The listing builds one solid part. Answer for the finished solid, in the listing's coordinates (mm). A direction names the side the tool comes from. Coordinates: 2 decimals unless noted, no trailing zeros. Loops run counter-clockwise (first coordinate to the right, second up) from the corner with the lowest first, then second, coordinate; pieces in that order, holes last. Notation, with made-up numbers: (43, 38) - (89, 38) arc R12 ccw to (89, 49) - close; hole circle Ø7 at (-8, -31.75). An arc over 180 degrees is marked (long way). Put each result on its own line as item: value.
```python
from build123d import *

# Parameters (mm, degrees)
F0_R     = 40.64
F0_R_2   = 33.02
F1_DEPTH = 152.4
F2_R     = 76.2
F3_DEPTH = 25.4
F4_R     = 5.08
F5_R     = 5.08


with BuildPart() as f1:
    # F0 (on Front) → F1 (new body)
    with BuildSketch(Plane.XZ):
        Circle(F0_R)
        Circle(F0_R_2, mode=Mode.SUBTRACT)
    extrude(amount=F1_DEPTH)

    # F2 (on Front) → F3 (join)
    with BuildSketch(Plane.XZ):
        Circle(F2_R)
    extrude(amount=-F3_DEPTH)

    # F4
    f4_edges = [f1.edges().sort_by_distance(p)[0] for p in [
        (76.2, 12.7, 0),
        (-76.2, 0, 0),
        (-76.2, 25.4, 0),
    ]]
    fillet(f4_edges, radius=F4_R)

    # F5
    f5_edges = [f1.edges().sort_by_distance(p)[0] for p in [
        (-40.64, -152.4, 0),
    ]]
    fillet(f5_edges, radius=F5_R)


solid = f1.part
```
1) Straight lines are drawn through the part: L1, parallel to Z at x = 0, y = -114; L2, parallel to Y at x = -10, z = -23.5; L3, parallel to Z at x = -6.5, y = -91.5. For each, find the intervals that lie inside material, in ascending order. Write a range as [from, to].
Found:
L1: z = [-40.64, -33.02], [33.02, 40.64]
L2: y = [0, 25.4]
L3: z = [-40.12, -32.37], [32.37, 40.12]
2) The part is cut by section B-B (z = 0). Give the vertices of the cut face in (x, y).
Found:
outline: (-76.2, 5.08) arc R5.08 ccw to (-71.12, 0) - (-40.64, 0) - (-40.64, -147.32) arc R5.08 ccw to (-35.56, -152.4) - (-33.02, -152.4) - (-33.02, 0) - (33.02, 0) - (33.02, -152.4) - (35.56, -152.4) arc R5.08 ccw to (40.64, -147.32) - (40.64, 0) - (71.12, 0) arc R5.08 ccw to (76.2, 5.08) - (76.2, 20.32) arc R5.08 ccw to (71.12, 25.4) - (-71.12, 25.4) arc R5.08 ccw to (-76.2, 20.32) - close
3) The part is cut by section C-C (y = -55.5). Give the vertices of the cut face in (x, z).
Found:
outline: circle Ø81.28 at (0, 0); hole circle Ø66.04 at (0, 0)
4) For a pull along Z with two mould halves and no side action, classify faces 1 (the face through (-60.47, 12.593, -46.367)), 2 (the face through (31.5, -75.1, 9.9)), 3 (the face through (31, 0, -31)) as pulls with the +Z half, pulls with the -Z half, needs draft (parallel to the pull), parting line crosses it, or undercut.
Found:
face 1: parting line crosses it
face 2: undercut
face 3: needs draft
5) The part is cut by section D-D (y = 14). Give the vertices of the cut face in (x, z), and give its area (3 significant figures).
Found:
outline: circle Ø152.4 at (0, 0)
area: 18,200 mm^2
6) For faces 4 (the face through (-1, 25.4, 1)), 5 (the face through (0, 0, 0)), determine the directions among +Z, -Z, +X, -X, +Y, -Y from which every point of the face is accessible in a straight line to the end or side of a thin tool.
Found:
face 4: +Z, -Z, +X, -X, +Y
face 5: -Y
7) Each of these flat-tipped pins is pushed along its axis until it touches: pin 1 (3 mm diameter, centred on x = -21.5, y = -19, fed in from +Z); pin 2 (10 mm diameter, centred on x = -59.5, z = 36, fed in from -Y); pin 3 (8 mm diameter, centred on y = -94, z = -14.5, fed in from -X). Where does it stop, or does it pass through?
Found:
pin 1: stops at z = 35.38
pin 2: stops at y = 0
pin 3: stops at x = -39.26
8) The part is cut by section A-A (x = 0). Give the vertices of the cut face in (y, z), and give its area (3 significant figures).
Found:
outline: (-152.4, -35.56) arc R5.08 ccw to (-147.32, -40.64) - (0, -40.64) - (0, -71.12) arc R5.08 ccw to (5.08, -76.2) - (20.32, -76.2) arc R5.08 ccw to (25.4, -71.12) - (25.4, 71.12) arc R5.08 ccw to (20.32, 76.2) - (5.08, 76.2) arc R5.08 ccw to (0, 71.12) - (0, 40.64) - (-147.32, 40.64) arc R5.08 ccw to (-152.4, 35.56) - (-152.4, 33.02) - (0, 33.02) - (0, -33.02) - (-152.4, -33.02) - close
area: 6,160 mm^2
